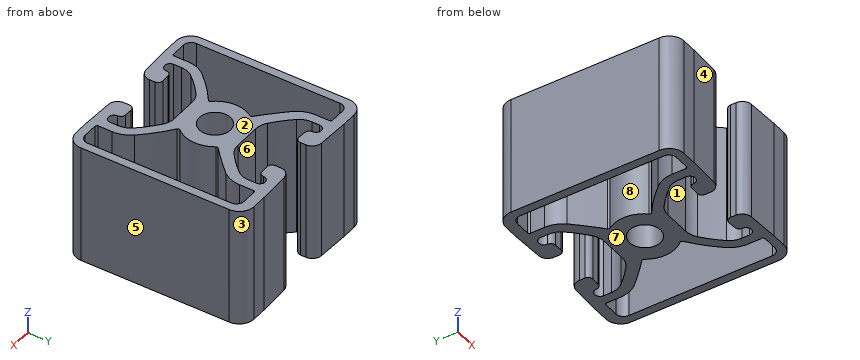
```python
from build123d import *

# Parameters (mm, degrees)
EXTRUDE1_DEPTH = 25.4


with BuildPart() as part:
    # Sketch1 → Extrude1 (new body)
    with BuildSketch(Plane.XY):
        with BuildLine():
            Line((119.286543537, 134.961539124), (116.458442746, 134.961539124))
            Line((116.458442746, 134.961539124), (113.630341955, 134.961539124))
            ThreePointArc((113.630341955, 134.961539124), (112.303785999, 135.184140252), (111.122551329, 135.827558172))
            ThreePointArc((111.122551329, 135.827558172), (109.143601343, 137.551745223), (107.353147508, 139.470947948))
            ThreePointArc((107.353147508, 139.470947948), (106.645746382, 140.694329655), (106.400042746, 142.085986537))
            Line((106.400042746, 142.085986537), (106.400042746, 143.768987481))
            ThreePointArc((106.400042746, 143.768987481), (107.548393057, 144.918338688), (108.698744289, 143.770990147))
            ThreePointArc((108.698744289, 143.770990147), (108.983276863, 143.067626667), (109.675740732, 142.757509334))
            Line((109.675740732, 142.757509334), (111.402940732, 142.691157003))
            ThreePointArc((111.402940732, 142.691157003), (112.146439004, 142.974328196), (112.457942746, 143.706408126))
            Line((112.457942746, 143.706408126), (112.457942746, 144.914700752))
            ThreePointArc((112.457942746, 144.914700752), (111.890102605, 146.323693267), (110.503946774, 146.945202999))
            Line((110.503946774, 146.945202999), (103.758442746, 147.204339124))
            Line((103.758442746, 147.204339124), (100.583442746, 147.204339124))
            ThreePointArc((100.583442746, 147.204339124), (98.338378716, 146.274403155), (97.408442746, 144.029339124))
            Line((97.408442746, 144.029339124), (97.408442746, 112.279339124))
            ThreePointArc((97.408442746, 112.279339124), (98.338378716, 110.034275094), (100.583442746, 109.104339124))
            Line((100.583442746, 109.104339124), (103.758442746, 109.104339124))
            Line((103.758442746, 109.104339124), (110.503946774, 109.36347525))
            ThreePointArc((110.503946774, 109.36347525), (111.890102605, 109.984984981), (112.457942746, 111.393977496))
            Line((112.457942746, 111.393977496), (112.457942746, 112.602270123))
            ThreePointArc((112.457942746, 112.602270123), (112.146439004, 113.334350053), (111.402940732, 113.617521246))
            Line((111.402940732, 113.617521246), (109.675740732, 113.551168915))
            ThreePointArc((109.675740732, 113.551168915), (108.983276863, 113.241051582), (108.698744289, 112.537688102))
            ThreePointArc((108.698744289, 112.537688102), (107.548393057, 111.390339561), (106.400042746, 112.539690768))
            Line((106.400042746, 112.539690768), (106.400042746, 114.222691712))
            ThreePointArc((106.400042746, 114.222691712), (106.645746382, 115.614348594), (107.353147508, 116.8377303))
            ThreePointArc((107.353147508, 116.8377303), (109.143601343, 118.756933026), (111.122551329, 120.481120077))
            ThreePointArc((111.122551329, 120.481120077), (112.303785999, 121.124537997), (113.630341955, 121.347139124))
            Line((113.630341955, 121.347139124), (116.458442746, 121.347139124))
            Line((116.458442746, 121.347139124), (119.286543537, 121.347139124))
            ThreePointArc((119.286543537, 121.347139124), (120.613099494, 121.124537997), (121.794334164, 120.481120077))
            ThreePointArc((121.794334164, 120.481120077), (123.77328415, 118.756933026), (125.563737985, 116.8377303))
            ThreePointArc((125.563737985, 116.8377303), (126.27113911, 115.614348594), (126.516842746, 114.222691712))
            Line((126.516842746, 114.222691712), (126.516842746, 112.539690768))
            ThreePointArc((126.516842746, 112.539690768), (125.368492436, 111.390339561), (124.218141204, 112.537688102))
            ThreePointArc((124.218141204, 112.537688102), (123.93360863, 113.241051582), (123.24114476, 113.551168915))
            Line((123.24114476, 113.551168915), (121.51394476, 113.617521246))
            ThreePointArc((121.51394476, 113.617521246), (120.770446489, 113.334350053), (120.458942746, 112.602270123))
            Line((120.458942746, 112.602270123), (120.458942746, 111.393977496))
            ThreePointArc((120.458942746, 111.393977496), (121.026782887, 109.984984981), (122.412938718, 109.36347525))
            Line((122.412938718, 109.36347525), (129.158442746, 109.104339124))
            Line((129.158442746, 109.104339124), (132.333442746, 109.104339124))
            ThreePointArc((132.333442746, 109.104339124), (134.578506777, 110.034275094), (135.508442746, 112.279339124))
            Line((135.508442746, 112.279339124), (135.508442746, 144.029339124))
            ThreePointArc((135.508442746, 144.029339124), (134.578506777, 146.274403155), (132.333442746, 147.204339124))
            Line((132.333442746, 147.204339124), (129.158442746, 147.204339124))
            Line((129.158442746, 147.204339124), (122.412938718, 146.945202999))
            ThreePointArc((122.412938718, 146.945202999), (121.026782887, 146.323693267), (120.458942746, 144.914700752))
            Line((120.458942746, 144.914700752), (120.458942746, 143.706408126))
            ThreePointArc((120.458942746, 143.706408126), (120.770446489, 142.974328196), (121.51394476, 142.691157003))
            Line((121.51394476, 142.691157003), (123.24114476, 142.757509334))
            ThreePointArc((123.24114476, 142.757509334), (123.93360863, 143.067626667), (124.218141204, 143.770990147))
            ThreePointArc((124.218141204, 143.770990147), (125.368492436, 144.918338688), (126.516842746, 143.768987481))
            Line((126.516842746, 143.768987481), (126.516842746, 142.085986537))
            ThreePointArc((126.516842746, 142.085986537), (126.27113911, 140.694329655), (125.563737985, 139.470947948))
            ThreePointArc((125.563737985, 139.470947948), (123.77328415, 137.551745223), (121.794334164, 135.827558172))
            ThreePointArc((121.794334164, 135.827558172), (120.613099494, 135.184140252), (119.286543537, 134.961539124))
        make_face()
        with BuildLine():
            Line((128.548842746, 141.559935312), (128.548842746, 144.5192879))
            ThreePointArc((128.548842746, 144.5192879), (128.660435063, 144.788695584), (128.929842746, 144.9002879))
            Line((128.929842746, 144.9002879), (132.079442746, 144.9002879))
            ThreePointArc((132.079442746, 144.9002879), (133.246876042, 144.416721196), (133.730442746, 143.2492879))
            Line((133.730442746, 143.2492879), (133.730442746, 112.533339124))
            ThreePointArc((133.730442746, 112.533339124), (133.246876042, 111.365905829), (132.079442746, 110.882339124))
            Line((132.079442746, 110.882339124), (128.929842746, 110.882339124))
            ThreePointArc((128.929842746, 110.882339124), (128.660435063, 110.993931441), (128.548842746, 111.263339124))
            Line((128.548842746, 111.263339124), (128.548842746, 114.222691712))
            ThreePointArc((128.548842746, 114.222691712), (128.180287293, 116.310177035), (127.119185604, 118.145249594))
            ThreePointArc((127.119185604, 118.145249594), (124.427739509, 120.92409139), (121.44277505, 123.384951196))
            ThreePointArc((121.44277505, 123.384951196), (121.277666857, 123.652597781), (121.370025317, 123.953206039))
            ThreePointArc((121.370025317, 123.953206039), (122.999396104, 127.891050115), (121.862557266, 131.998246553))
            ThreePointArc((121.862557266, 131.998246553), (121.797364551, 132.248793719), (121.907342287, 132.483162808))
            ThreePointArc((121.907342287, 132.483162808), (124.57297323, 134.999893232), (127.119185604, 137.63737743))
            ThreePointArc((127.119185604, 137.63737743), (128.180287293, 139.47244999), (128.548842746, 141.559935312))
        make_face(mode=Mode.SUBTRACT)
        with BuildLine():
            Line((104.368042746, 141.559935312), (104.368042746, 144.5192879))
            ThreePointArc((104.368042746, 144.5192879), (104.25645043, 144.788695584), (103.987042746, 144.9002879))
            Line((103.987042746, 144.9002879), (100.837442746, 144.9002879))
            ThreePointArc((100.837442746, 144.9002879), (99.670009451, 144.416721196), (99.186442746, 143.2492879))
            Line((99.186442746, 143.2492879), (99.186442746, 112.533339124))
            ThreePointArc((99.186442746, 112.533339124), (99.670009451, 111.365905829), (100.837442746, 110.882339124))
            Line((100.837442746, 110.882339124), (103.987042746, 110.882339124))
            ThreePointArc((103.987042746, 110.882339124), (104.25645043, 110.993931441), (104.368042746, 111.263339124))
            Line((104.368042746, 111.263339124), (104.368042746, 114.222691712))
            ThreePointArc((104.368042746, 114.222691712), (104.7365982, 116.310177035), (105.797699889, 118.145249594))
            ThreePointArc((105.797699889, 118.145249594), (108.489145984, 120.92409139), (111.474110443, 123.384951196))
            ThreePointArc((111.474110443, 123.384951196), (111.639218636, 123.652597781), (111.546860176, 123.953206039))
            ThreePointArc((111.546860176, 123.953206039), (109.917489388, 127.891050115), (111.054328227, 131.998246553))
            ThreePointArc((111.054328227, 131.998246553), (111.119520942, 132.248793719), (111.009543206, 132.483162808))
            ThreePointArc((111.009543206, 132.483162808), (108.343912263, 134.999893232), (105.797699889, 137.63737743))
            ThreePointArc((105.797699889, 137.63737743), (104.7365982, 139.47244999), (104.368042746, 141.559935312))
        make_face(mode=Mode.SUBTRACT)
        with BuildLine():
            ThreePointArc((116.458442746, 131.456339124), (113.156442746, 128.154339124), (116.458442746, 124.852339124))
            ThreePointArc((116.458442746, 124.852339124), (119.760442746, 128.154339124), (116.458442746, 131.456339124))
        make_face(mode=Mode.SUBTRACT)
    extrude(amount=EXTRUDE1_DEPTH)


solid = part.part
```
The model under review builds one solid part; all positions refer to its coordinate system, in mm. Face numbers are marked on the shaded views. A direction names the side the tool comes from. Round coordinates to 2 decimals unless told otherwise and drop trailing zeros. Loops run counter-clockwise (first coordinate to the right, second up) from the corner with the lowest first, then second, coordinate; pieces in that order, holes last.
Item 1: Take a section at B-B (x = 128). Write out the cut boundary in (y, z), then the cut area to 3 significant figures.
Determined:
outline: (109.15, 0) - (116.75, 0) - (116.75, 25.4) - (109.15, 25.4) - close; (139.03, 0) - (147.16, 0) - (147.16, 25.4) - (139.03, 25.4) - close
area: 400 mm2
Item 2: Mouldability with a two-part tool opening along X and no side actions: class the marked faces 1, 2 and 3 as released by +X, released by -X, zero draft, split by the parting line, or undercut.
Determined:
face 1: undercut
face 2: zero draft
face 3: released by +X
Item 3: Take a section at C-C (y = 133.5). Write out the cut boundary in (x, z), then the cut area to 3 significant figures.
Determined:
outline: (97.41, 0) - (99.19, 0) - (99.19, 25.4) - (97.41, 25.4) - close; (109.9, 0) - (123.01, 0) - (123.01, 25.4) - (109.9, 25.4) - close; (133.73, 0) - (135.51, 0) - (135.51, 25.4) - (133.73, 25.4) - close
area: 423 mm2
Item 4: Clearance check with flat-ended pins moving along their axes: pin 1 Ø3 at (x, z) = (117, 16) entering from +Y; pin 2 Ø1.5 at (x, z) = (113.5, 18.5) entering from +Y; pin 3 Ø6 at (x, z) = (117, 10.5) entering from -Y. State where each tip first meets the part, or that it passes through.
Determined:
pin 1: stops at y = 134.96
pin 2: stops at y = 135.06
pin 3: stops at y = 121.28
Item 5: For the marked faces 4, 5, 6, 7 and 8, list the 3-axis set-ups (+Z, -Z, +X, -X, +Y, -Y) from which the entire face can be reached by the end or side of a thin tool; tool diameter is ignored.
Determined:
face 4: +Z, -Z, -Y
face 5: +Z, -Z, +X, +Y, -Y
face 6: +Z, -Z, +Y
face 7: -Z, +X, -X, +Y, -Y
face 8: +Z, -Z
Item 6: Take a section at D-D (z = 21.75). Give the number of separate pieces and of enclosed holes in the cut face, then the cut area to 3 significant figures.
Determined:
separate pieces: 1
enclosed holes: 3
area: 506 mm2
Item 7: Take a section at A-A (y = 125.5). Write out the cut boundary in (x, z), then the cut area to 3 significant figures.
Determined:
outline: (97.41, 0) - (99.19, 0) - (99.19, 25.4) - (97.41, 25.4) - close; (110.53, 0) - (114.49, 0) - (114.49, 25.4) - (110.53, 25.4) - close; (118.42, 0) - (122.39, 0) - (122.39, 25.4) - (118.42, 25.4) - close; (133.73, 0) - (135.51, 0) - (135.51, 25.4) - (133.73, 25.4) - close
area: 292 mm2
Item 8: For line 1 (X direction, y = 114, z = 18.25); line 2 (Y direction, x = 131, z = 21.25); line 3 (X direction, y = 134.5, z = 7.5), list the stretches that pass through material, from the lowest coordinate up.
Determined:
line 1: x = 97.41 to 99.19, 104.37 to 106.4, 126.52 to 128.55, 133.73 to 135.51
line 2: y = 109.1 to 110.88, 144.9 to 147.2
line 3: x = 97.41 to 99.19, 108.85 to 124.06, 133.73 to 135.51
